Could you check a few things on this model? Use its own coordinates, in mm. Face numbers are marked on the shaded views. Give positions to 0.01 mm unless a question says otherwise; leave off trailing zeros. Loops run counter-clockwise (first coordinate to the right, second up) from the corner with the lowest first, then second, coordinate; pieces in that order, holes last. Notation, with made-up numbers: M -35.5,-5.5 L -20.5,-5.5 A35 ccw -20.5,30.5 Z; hole C -15.5,22.25 d7. An arc over 180 degrees is marked long. Use a Markdown table: item, result. Add a question column.
1) Will these pins go through, and if not, where does the flat tip stop? pin 1 Ø1.5 at (x, z) = (-48.5, 2) entering from +Y; pin 2 Ø10 at (x, y) = (19, -36) entering from +Z; pin 3 Ø3 at (x, y) = (29.43, -36.5) entering from -Z; pin 4 Ø2 at (y, z) = (-38, 4) entering from +X.
2) Suppose I cut it at B-B on z = 0.95. List the corners of the cut face in (x, y) for me, and give its area (3 significant figures).
3) We'd pull the mould along X, two halves only. Please class the marked faces 1, 2 and 3: +X half, -X half, draft (parallel to the pull), parting line (faces both ways), or undercut.
4) If I drill on line 1 along X through (y, z) = (-36.5, 2.9); line 2 along X through (y, z) = (-44.75, 2.1); line 3 along X through (y, z) = (-36.5, 3.5), over which ranges is the centre line in solid material (lowest first)? Write a range as [from, to].
5) Suppose I cut it at D-D on x = -21. List the corners of the cut face in (y, z) for me, and give its area (3 significant figures).
6) Suppose I cut it at A-A on y = -47. List the corners of the cut face in (x, z) for me, and give its area (3 significant figures).
7) Suppose I cut it at C-C on x = 46.5. List the corners of the cut face in (y, z) for me.
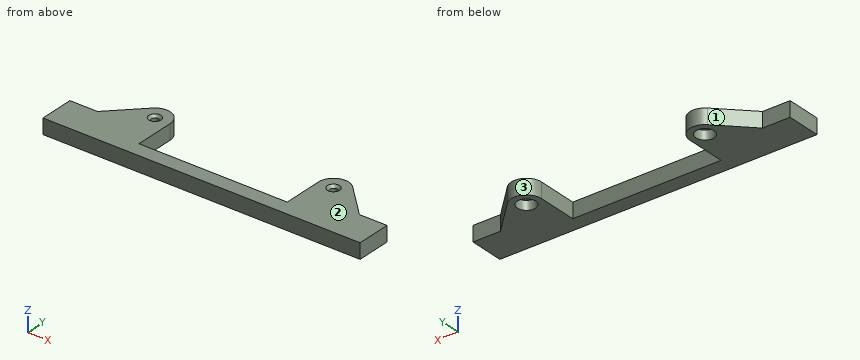
```python
from build123d import *

# Parameters (mm, degrees)
PAD_DEPTH        = 5
SKETCH_R         = 3
POCKET_DEPTH     = 3
HOLE_D           = 2.4
HOLE_CSINK_D     = 4
HOLE_CSINK_ANGLE = 90


with BuildPart() as part:
    # Sketch_1 → Pad (new body)
    with BuildSketch(Plane.XY):
        with BuildLine():
            ThreePointArc((-24.428932, -36.5), (-27.515515, -31.880602), (-32.964466, -32.964466))
            Line((-43.16455, -43.16455), (-32.964466, -32.964466))
            Line((-43.16455, -43.16455), (-52.247863, -43.16455))
            Line((-52.247863, -43.16455), (-52.247863, -54.512786))
            Line((-52.247863, -54.512786), (52.247863, -54.512786))
            Line((52.247863, -43.16455), (52.247863, -54.512786))
            Line((43.16455, -43.16455), (52.247863, -43.16455))
            Line((32.964466, -32.964466), (43.16455, -43.16455))
            ThreePointArc((32.964466, -32.964466), (27.515515, -31.880602), (24.428932, -36.5))
            Line((24.428932, -36.5), (24.428932, -49.634615))
            Line((-24.428932, -49.634615), (24.428932, -49.634615))
            Line((-24.428932, -36.5), (-24.428932, -49.634615))
        make_face()
    extrude(amount=PAD_DEPTH)

    # Sketch (on Face13 of Pad) → Pocket (cut)
    with BuildSketch(Plane(origin=(0, 0, 0), x_dir=(1, 0, 0), z_dir=(0, 0, -1))):
        with Locations((-29.428932, 36.5)):
            Circle(SKETCH_R)
        with Locations((29.428932, 36.5)):
            Circle(SKETCH_R)
    extrude(amount=-POCKET_DEPTH, mode=Mode.SUBTRACT)

    # Hole (through all)
    with Locations(Plane.XY.offset(5)):
        with Locations((-29.428932, -36.5), (29.428932, -36.5)):
            CounterSinkHole(HOLE_D / 2, HOLE_CSINK_D / 2, counter_sink_angle=HOLE_CSINK_ANGLE)


solid = part.part
```
Answer block:
| question | item | result |
|---|---|---|
| 1 | pin 1 | stops at y = -43.16 |
| 1 | pin 2 | passes through |
| 1 | pin 3 | stops at z = 3 |
| 1 | pin 4 | stops at x = 39 |
| 2 | outline | M -52.25,-54.51 L 52.25,-54.51 L 52.25,-43.16 L 43.16,-43.16 L 32.96,-32.96 A5 ccw 24.43,-36.5 L 24.43,-49.63 L -24.43,-49.63 L -24.43,-36.5 A5 ccw -32.96,-32.96 L -43.16,-43.16 L -52.25,-43.16 Z; hole C -29.43,-36.5 d6; hole C 29.43,-36.5 d6 |
| 2 | area | 1,100 mm^2 |
| 3 | face 1 | -X half |
| 3 | face 2 | draft |
| 3 | face 3 | undercut |
| 4 | line 1 | x = [-36.5, -32.43], [-26.43, -24.43], [24.43, 26.43], [32.43, 36.5] |
| 4 | line 2 | x = [-52.25, -24.43], [24.43, 52.25] |
| 4 | line 3 | x = [-36.5, -30.63], [-28.23, -24.43], [24.43, 28.23], [30.63, 36.5] |
| 5 | outline | M -54.51,0 L -49.63,0 L -49.63,5 L -54.51,5 Z |
| 5 | area | 24.4 mm^2 |
| 6 | outline | M -52.25,0 L -24.43,0 L -24.43,5 L -52.25,5 Z; M 24.43,0 L 52.25,0 L 52.25,5 L 24.43,5 Z |
| 6 | area | 278 mm^2 |
| 7 | outline | M -54.51,0 L -43.16,0 L -43.16,5 L -54.51,5 Z |
